```python
from build123d import *

# Parameters (mm, degrees)
ESQUISSE1_W        = 25
ESQUISSE1_H        = 25
ESQUISSE1_W_2      = 21
ESQUISSE1_H_2      = 21
BOSS_EXTRU_1_DEPTH = 30
ESQUISSE2_W        = 37
ESQUISSE2_H        = 37
ESQUISSE2_W_2      = 25
ESQUISSE2_H_2      = 25
BOSS_EXTRU_2_DEPTH = 5
CONG_1_R           = 10
CONG_2_R           = 3


with BuildPart() as part:
    # Esquisse1 → Boss.-Extru.1 (new body)
    with BuildSketch(Plane.XY):
        Rectangle(ESQUISSE1_W, ESQUISSE1_H)
        Rectangle(ESQUISSE1_W_2, ESQUISSE1_H_2, mode=Mode.SUBTRACT)
    extrude(amount=BOSS_EXTRU_1_DEPTH)

    # Esquisse2 → Boss.-Extru.2 (add)
    with BuildSketch(Plane.XY.offset(30)):
        Rectangle(ESQUISSE2_W, ESQUISSE2_H)
        Rectangle(ESQUISSE2_W_2, ESQUISSE2_H_2, mode=Mode.SUBTRACT)
    extrude(amount=-BOSS_EXTRU_2_DEPTH)

    # Congé1
    cong_1_edges = [part.edges().sort_by_distance(p)[0] for p in [
        (18.5, -18.5, 27.5),
        (-18.5, -18.5, 27.5),
        (-18.5, 18.5, 27.5),
        (18.5, 18.5, 27.5),
    ]]
    fillet(cong_1_edges, radius=CONG_1_R)

    # Congé2
    cong_2_edges = [part.edges().sort_by_distance(p)[0] for p in [
        (12.5, -12.5, 12.5),
        (-12.5, -12.5, 12.5),
        (-12.5, 12.5, 12.5),
        (12.5, 12.5, 12.5),
    ]]
    fillet(cong_2_edges, radius=CONG_2_R)


solid = part.part
```
Here's how the part is built. I have some questions about the finished solid (model axes, mm). A direction names the side the tool comes from. Round coordinates to 2 decimals unless told otherwise and drop trailing zeros. Loops run counter-clockwise (first coordinate to the right, second up) from the corner with the lowest first, then second, coordinate; pieces in that order, holes last.
1. Suppose I cut it at A-A, the plane y = -6. Please give me the cut outline in (x, z), and give its area (3 significant figures).
Answers:
outline: (-18.5, 25) - (-12.5, 25) - (-12.5, 0) - (-10.5, 0) - (-10.5, 30) - (-18.5, 30) - close; (10.5, 0) - (12.5, 0) - (12.5, 25) - (18.5, 25) - (18.5, 30) - (10.5, 30) - close
area: 180 mm2
2. Suppose I cut it at D-D, the plane y = 11. Please give me the cut outline in (x, z).
Answers:
outline: (-18.18, 25) - (-12.1, 25) - (-12.1, 0) - (12.1, 0) - (12.1, 25) - (18.18, 25) - (18.18, 30) - (-18.18, 30) - close
3. Suppose I cut it at B-B, the plane z = 22.75. Please give me the cut outline in (x, y).
Answers:
outline: (-12.5, -9.5) arc R3 ccw to (-9.5, -12.5) - (9.5, -12.5) arc R3 ccw to (12.5, -9.5) - (12.5, 9.5) arc R3 ccw to (9.5, 12.5) - (-9.5, 12.5) arc R3 ccw to (-12.5, 9.5) - close; hole (-10.5, -10.5) - (10.5, -10.5) - (10.5, 10.5) - (-10.5, 10.5) - close
4. If I drill on probe 1 along X at (y, z) = (6.5, 18); probe 2 along X at (y, z) = (-8, 28.25), over which ranges is the centre line in solid material (lowest first)?
Answers:
probe 1: x = -12.5 to -10.5, 10.5 to 12.5
probe 2: x = -18.5 to -10.5, 10.5 to 18.5
5. For faces 1 (the face through (0, 12.5, 12)), 2 (the face through (-11.6, -11.64, 12.68)), 3 (the face through (0, 10.5, 15)), 4 (the face through (12.5, 0, 12)), which set-ups out of +Z, -Z, +X, -X, +Y, -Y let a thin tool reach every point of the face, with its end or its side?
Answers:
face 1: -Z, +X, -X, +Y
face 2: -Z, -X, -Y
face 3: +Z, -Z
face 4: -Z, +X, +Y, -Y
6. Thinking about a two-plate mould opening in Y: for faces 5 (the face through (11.6, -11.64, 12.68)), 6 (the face through (0, -10.5, 15)), 7 (the face through (-11, 0, 0)), which applies, released by +Y, released by -Y, zero draft, split by the parting line, or undercut?
Answers:
face 5: released by -Y
face 6: undercut
face 7: zero draft
7. Will these pins go through, and if not, where does the flat tip stop? pin 1 (1.5 mm diameter, centred on y = 0, z = 19.5, fed in from +X); pin 2 (1 mm diameter, centred on y = -11, z = 9, fed in from +X); pin 3 (10.5 mm diameter, centred on y = 3, z = 13.5, fed in from -X); pin 4 (8 mm diameter, centred on x = 3, y = -1, fed in from +Z).
Answers:
pin 1: stops at x = 12.5
pin 2: stops at x = 12.33
pin 3: stops at x = -12.5
pin 4: passes through
